Could you check a few things on this model? Use its own coordinates, in mm. A direction names the side the tool comes from. Coordinates: 2 decimals unless noted, no trailing zeros. Loops run counter-clockwise (first coordinate to the right, second up) from the corner with the lowest first, then second, coordinate; pieces in that order, holes last.
from build123d import *

# Parameters (mm, degrees)
SKETCH_1_R      = 8.75
SKETCH_1_R_2    = 8
EXTRUDE_1_DEPTH = 175
SKETCH_2_W      = 20
SKETCH_2_H      = 20
EXTRUDE_2_DEPTH = 25
SKETCH_3_W      = 20
SKETCH_3_H      = 20
SKETCH_3_R      = 4
EXTRUDE_3_DEPTH = 15
FILLET_1_R      = 5
SKETCH_5_R      = 5
SKETCH_5_R_2    = 2.212387265
EXTRUDE_4_DEPTH = 10


with BuildPart() as part:
    # 草图1 → 凸台-拉伸1 (new body)
    with BuildSketch(Plane.XY):
        Circle(SKETCH_1_R)
        Circle(SKETCH_1_R_2, mode=Mode.SUBTRACT)
    extrude(amount=EXTRUDE_1_DEPTH)

    # 草图2 → 凸台-拉伸2 (add)
    with BuildSketch(Plane.XY):
        Rectangle(SKETCH_2_W, SKETCH_2_H)
    extrude(amount=EXTRUDE_2_DEPTH)

    # 草图3 → 凸台-拉伸3 (add)
    with BuildSketch(Plane.XY.offset(175)):
        Rectangle(SKETCH_3_W, SKETCH_3_H)
        Circle(SKETCH_3_R, mode=Mode.SUBTRACT)
    extrude(amount=-EXTRUDE_3_DEPTH)

    # 圆角1
    fillet_1_edges = [part.edges().sort_by_distance(p)[0] for p in [
        (10, -10, 12.5),
        (10, 10, 12.5),
        (-10, 10, 12.5),
        (-10, -10, 12.5),
        (10, -10, 167.5),
        (-10, -10, 167.5),
        (-10, 10, 167.5),
        (10, 10, 167.5),
    ]]
    fillet(fillet_1_edges, radius=FILLET_1_R)

    # 草图5 → 凸台-拉伸4 (add)
    with BuildSketch(Plane.XY.offset(175)):
        Circle(SKETCH_5_R)
        Circle(SKETCH_5_R_2, mode=Mode.SUBTRACT)
    extrude(amount=EXTRUDE_4_DEPTH)


solid = part.part
(1) We'd pull the mould along X, two halves only. Please class faces 1 (the face through (2.1, 0.7, 179.9)), 2 (the face through (0, -10, 168)), 3 (the face through (10, 0, 168)): +X half, -X half, draft (parallel to the pull), parting line (faces both ways), or undercut.
Answers:
face 1: undercut
face 2: draft
face 3: +X half
(2) For pin 1 (5 mm diameter, centred on x = -3, z = 91, fed in from +Y); pin 2 (10 mm diameter, centred on y = -5.5, z = 118, fed in from -X); pin 3 (2.5 mm diameter, centred on x = 0, y = 0, fed in from +Z), each with a flat end and sliding along its axis, tell me the tip position at first contact or that it passes through.
Answers:
pin 1: stops at y = 8.74
pin 2: stops at x = -8.74
pin 3: stops at z = 25
(3) Imagine slicing it at A-A, the plane x = 0. Write out the boundary of the cut face in (y, z), and give its area (3 significant figures).
Answers:
outline: (-10, 0) - (10, 0) - (10, 25) - (8.75, 25) - (8.75, 160) - (10, 160) - (10, 175) - (5, 175) - (5, 185) - (2.21, 185) - (2.21, 175) - (4, 175) - (4, 160) - (8, 160) - (8, 25) - (-8, 25) - (-8, 160) - (-4, 160) - (-4, 175) - (-2.21, 175) - (-2.21, 185) - (-5, 185) - (-5, 175) - (-10, 175) - (-10, 160) - (-8.75, 160) - (-8.75, 25) - (-10, 25) - close
area: 938 mm2
(4) I need wall thicknesses on probe 1 along Z at (x, y) = (6.75, -9); probe 2 along Y at (x, z) = (0, 169); probe 3 along Y at (x, z) = (0, 177.75). Which ranges of each line are inside material? Lowest first, please.
Answers:
probe 1: z = 0 to 25, 160 to 175
probe 2: y = -10 to -4, 4 to 10
probe 3: y = -5 to -2.21, 2.21 to 5
(5) Imagine slicing it at C-C, the plane z = 112. Write out the boundary of the cut face in (x, y), and give its area (3 significant figures).
Answers:
outline: circle Ø17.5 at (0, 0); hole circle Ø16 at (0, 0)
area: 39.5 mm2
(6) Which directions (+Z, -Z, +X, -X, +Y, -Y) give clear straight access to the entire face, cutting with the end or side of a thin tool? Please do faces 4 (the face through (2, -2, 175)), 5 (the face through (8, 9, 167)), 6 (the face through (-1.08, -4.88, 179.93)).
Answers:
face 4: none
face 5: +Z, -Z, +X, +Y
face 6: +Z
